For this review, take the finished solid that the model builds, in its own axes (mm). A direction names the side the tool comes from. Coordinates: 2 decimals unless noted, no trailing zeros. Write each loop counter-clockwise with the first axis right and the second up, starting at its lowest first coordinate (ties: lowest second). Pieces come first, ordered by that corner, then holes.
```python
from build123d import *

# Parameters (mm, degrees)
SKETCH1_W           = 330.2
SKETCH1_H           = 12.7
BOSS_EXTRUDE1_DEPTH = 50.8
CUT_EXTRUDE1_REACH  = 336.145
FILLET1_R           = 2.54


with BuildPart() as part:
    # Sketch1 → Boss-Extrude1 (new body)
    with BuildSketch(Plane.XY):
        Rectangle(SKETCH1_W, SKETCH1_H)
    extrude(amount=BOSS_EXTRUDE1_DEPTH)

    # Sketch2 → Cut-Extrude1 (cut, up to next)
    with BuildSketch(Plane.ZY.offset(165.1), mode=Mode.PRIVATE) as cut_extrude1_sk1:
        Polygon((41.27098203, -6.35), (41.27098203, -4.509591524), (39.332279131, -4.509591524), (39.332279131, -1.969591524), (45.749684928, -1.969591524), (45.749684928, -4.509591524), (43.81098203, -4.509591524), (43.81098203, -6.35), align=None)
    cut_extrude1_tool1 = extrude(cut_extrude1_sk1.sketch, amount=-CUT_EXTRUDE1_REACH, mode=Mode.PRIVATE) & part.part
    cut_extrude1 = cut_extrude1_tool1.solids().sort_by_distance((-165.1, -3.72772, 42.540982))[0]
    add(cut_extrude1, mode=Mode.SUBTRACT)

    # Mirror1: Cut-Extrude1 across plane
    add(cut_extrude1.mirror(Plane.XY.offset(25.4)), mode=Mode.SUBTRACT)

    # Fillet1
    fillet1_edges = [part.edges().sort_by_distance(p)[0] for p in [
        (0, 6.35, 50.8),
        (0, 6.35, 0),
        (0, -6.35, 0),
        (0, -6.35, 50.8),
    ]]
    fillet(fillet1_edges, radius=FILLET1_R)


solid = part.part
```
Q1. For probe 1 along Y at (x, z) = (100, 6); probe 2 along Z at (x, y) = (-126.5, -2); probe 3 along Z at (x, y) = (33, -5.5), list the stretches that pass through material, from the lowest coordinate up.
Ans:
probe 1: y = -6.35 to -4.51, -1.97 to 6.35
probe 2: z = 0 to 5.05, 11.47 to 39.33, 45.75 to 50.8
probe 3: z = 0.64 to 6.99, 9.53 to 41.27, 43.81 to 50.16
Q2. Add section A-A (x = 54.5). State the section outline as (y, z) points, then the cut area to 3 significant figures.
Ans:
outline: (-6.35, 2.54) arc R2.54 ccw to (-3.81, 0) - (3.81, 0) arc R2.54 ccw to (6.35, 2.54) - (6.35, 48.26) arc R2.54 ccw to (3.81, 50.8) - (-3.81, 50.8) arc R2.54 ccw to (-6.35, 48.26) - (-6.35, 43.81) - (-4.51, 43.81) - (-4.51, 45.75) - (-1.97, 45.75) - (-1.97, 39.33) - (-4.51, 39.33) - (-4.51, 41.27) - (-6.35, 41.27) - (-6.35, 9.53) - (-4.51, 9.53) - (-4.51, 11.47) - (-1.97, 11.47) - (-1.97, 5.05) - (-4.51, 5.05) - (-4.51, 6.99) - (-6.35, 6.99) - close
area: 598 mm2
Q3. Tool access review of faces 5 (the flat face through (-2, -1.97, 42)), 6 (the flat face through (-2, 6.35, 25)): name each direction out of +Z, -Z, +X, -X, +Y, -Y from which nothing blocks a thin tool from reaching the whole face with its end or side.
Ans:
face 5: +X, -X
face 6: +Z, -Z, +X, -X, +Y
Q4. Clearance check with flat-ended pins moving along their axes: pin 1 Ø2 at (x, y) = (-17.5, -5) entering from -Z; pin 2 Ø0.9 at (x, y) = (76.5, -5.5) entering from -Z; pin 3 Ø0.6 at (x, y) = (-48, -5.5) entering from +Z. State where each tip first meets the part, or that it passes through.
Ans:
pin 1: stops at z = 0.01
pin 2: stops at z = 0.32
pin 3: stops at z = 50.39
Q5. Draft analysis for pull direction Z (two halves, no side actions). For faces 1 (the flat face through (-2, 0, 0)), 2 (the flat face through (-165.1, 0, 25)), 3 (the flat face through (-2, -1.97, 8)), 4 (the flat face through (-2, 0, 50.8)), state which applies: +Z half, -Z half, draft (parallel to the pull), parting line (faces both ways), or undercut.
Ans:
face 1: -Z half
face 2: draft
face 3: undercut
face 4: +Z half
